from build123d import *

# Parameters (mm, degrees)
F2_R     = 2.5
F4_DEPTH = 5
F5_COUNT = 12
F5_ANGLE = 330
F6_R     = 7.8035714286
F6_R_2   = 5
F7_DEPTH = 1.5
F8_START = 3.5
F8_DEPTH = 1.5


# Not quite as in the source:
# - a feature names something its author has since deleted; it is built from what else it names


with BuildPart() as f4:
    # F2 (on Top) → F4 (new body)
    with BuildSketch(Plane.XY):
        with BuildLine():
            ThreePointArc((-2.828404167, 9.9077602944), (-1.3448859448, 10.2154229467), (0.1677115736, 10.3022064147))
            ThreePointArc((0.1677115736, 10.3022064147), (0.1151870939, 12.4936954813), (-0.981879075, 14.3915439923))
            Line((-0.981879075, 14.3915439923), (-2.7763833168, 14.1552930269))
            ThreePointArc((-2.7763833168, 14.1552930269), (-3.3448685232, 12.0381705175), (-2.828404167, 9.9077602944))
        make_face()
        with BuildLine():
            ThreePointArc((-2.828404167, 9.9077602944), (-6.2056796493, -8.2251519301), (10.3035714286, 0))
            ThreePointArc((10.3035714286, 0), (7.3447808804, 7.2261869615), (0.1677115736, 10.3022064147))
            ThreePointArc((0.1677115736, 10.3022064147), (-1.3448859448, 10.2154229467), (-2.828404167, 9.9077602944))
        make_face()
        Circle(F2_R, mode=Mode.SUBTRACT)
    extrude(amount=F4_DEPTH)

    # F5: F4 ×12 about axis
    f5_axis = Axis((0, 0, 30.7848658413), (0, 0, 1))


with BuildPart() as f4_1:
    add(f4.part)
    for i in range(1, F5_COUNT):
        add(f4.part.rotate(f5_axis, i * F5_ANGLE / (F5_COUNT - 1)))

    # F6 (on Top) → F7 (cut)
    with BuildSketch(Plane.XY):
        Circle(F6_R)
        Circle(F6_R_2, mode=Mode.SUBTRACT)
    extrude(amount=F7_DEPTH, mode=Mode.SUBTRACT)

    # F6 (on Top) → F8 (cut)
    with BuildSketch(Plane.XY.offset(F8_START)):
        Circle(F6_R)
        Circle(F6_R_2, mode=Mode.SUBTRACT)
    extrude(amount=F8_DEPTH, mode=Mode.SUBTRACT)


solid = f4_1.part
Model file for the job. Use its own axes, mm. A direction names the side the tool comes from. Give positions to 0.01 mm unless a question says otherwise; leave off trailing zeros. Order: outer loops, then holes, each group sorted by start corner. A loop starts at its lowest first (then second) coordinate and runs counter-clockwise, first axis right, second up. Notation, with made-up numbers: (66, 20) - (110, 20) arc R25 cw to (110, 42) - close; hole circle Ø3 at (9.25, 60). An arc over 180 degrees is marked (long way). One line per item, written item: value.
Item 1: Two-plate mould, pull along X, no slides. Class faces 1 (the flat face through (1.867, -14.275, 2.465)), 2 (the cylindrical face through (12.069, 3.344, 2.465)), 3 (the flat face through (-3, 0, 0)): released by +X, released by -X, zero draft, split by the parting line, or undercut.
Response values:
face 1: released by +X
face 2: undercut
face 3: zero draft
Item 2: Pin check, flat tip, straight feed: pin 1 Ø1 at (y, z) = (1, 0.5) entering from -X. Stop position of the tip, or through.
Response values:
pin 1: x = -10.29
Item 3: Slice it at B-B (z = 4.5). Give the number of separate pieces and of enclosed holes in the cut face, then the cut area to 3 significant figures.
Response values:
separate pieces: 2
enclosed holes: 2
area: 358 mm2
Item 4: Slice it at D-D (y = -1.5). List the corners of the cut face in (x, z).
Response values:
outline: (-14.32, 0) - (-7.66, 0) - (-7.66, 1.5) - (-4.77, 1.5) - (-4.77, 0) - (-2, 0) - (-2, 5) - (-4.77, 5) - (-4.77, 3.5) - (-7.66, 3.5) - (-7.66, 5) - (-14.32, 5) - close; (2, 0) - (4.77, 0) - (4.77, 1.5) - (7.66, 1.5) - (7.66, 0) - (10.19, 0) - (10.19, 5) - (7.66, 5) - (7.66, 3.5) - (4.77, 3.5) - (4.77, 5) - (2, 5) - close
Item 5: Slice it at C-C (x = 11.5). List the corners of the cut face in (y, z).
Response values:
outline: (-6.47, 0) - (-2.83, 0) - (-2.83, 5) - (-6.47, 5) - close; (-0.28, 0) - (3.32, 0) - (3.32, 5) - (-0.28, 5) - close; (6.95, 0) - (8.66, 0) - (8.66, 5) - (6.95, 5) - close
Item 6: Tool access for faces 4 (the flat face through (-8.75, 11.43, 2.46)), 5 (the flat face through (5, -2, 3.5)): list every direction of +Z, -Z, +X, -X, +Y, -Y with a clear straight run to the whole face (end or side of a thin tool).
Response values:
face 4: +Z, -Z, -X, +Y
face 5: +Z
Item 7: Slice it at A-A (y = 11.25). List the corners of the cut face in (x, z).
Response values:
outline: (-8.99, 0) - (-6.58, 0) - (-6.58, 5) - (-8.99, 5) - close; (-3.28, 0) - (0.28, 0) - (0.28, 5) - (-3.28, 5) - close; (2.73, 0) - (6.44, 0) - (6.44, 5) - (2.73, 5) - close
Item 8: Wall check: line 1 (Y direction, x = -11.5, z = 2.65); line 2 (Y direction, x = 13, z = 1.4); line 3 (Y direction, x = -12.5, z = 1.1). Give the ranges that are in metal, low to high.
Response values:
line 1: -8.66 to -6.95, -3.32 to 0.28, 2.83 to 6.47
line 2: -6.24 to -3.83, 0.06 to 3.23
line 3: -3.32 to 0.11, 3.39 to 6.44
